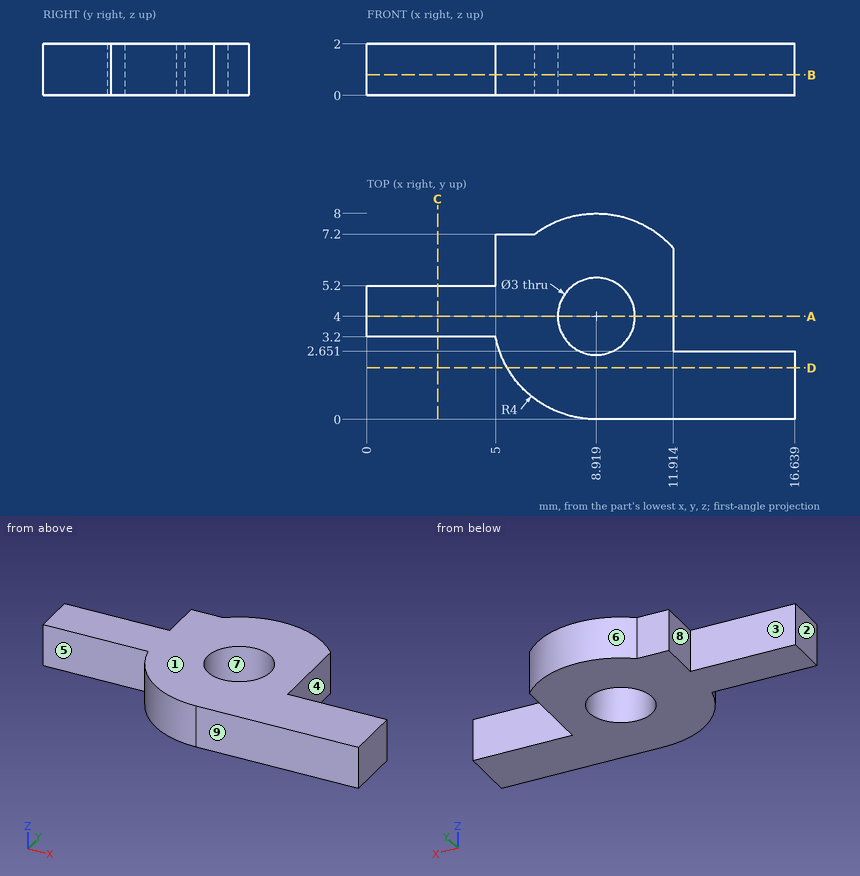
Geometry: see drawing. Coordinates: mm, zero at the bounding-box minimum. A direction names the side the tool comes from. Round coordinates to 2 decimals unless told otherwise and drop trailing zeros. Write each loop counter-clockwise with the first axis right and the second up, starting at its lowest first coordinate (ties: lowest second). Pieces come first, ordered by that corner, then holes.
Item 1: Mould query, pull axis Y, two halves, no side actions, for the marked faces 6, 7, 8 and 9. Classes: +Y half, -Y half, draft (parallel to the pull), parting line (faces both ways), or undercut.
Item 2: Material intervals for L1, parallel to X at y = 6.5, z = 0.75 (1 decimal); L2, parallel to Y at x = 4.75, z = 1.35; L3, parallel to Y at x = 14.25, z = 1.65, sorted ascending.
Item 3: Section query C-C (x = 2.75). Return loops of the section in (y, z).
Item 4: Set-up query: the marked faces 1, 2, 3, 4 and 5. Return all of +Z, -Z, +X, -X, +Y, -Y with unobstructed straight access to the full face (end or side cutting, diameter ignored); none if empty.
Item 5: Section query D-D (y = 2). Return loops of the section in (x, z) (1 decimal).
Item 6: Section query A-A (y = 4). Return loops of the section in (x, z) (1 decimal).
Item 7: Section query B-B (z = 0.8). Return loops of the section in (x, y) (1 decimal).
Item 8: Pin query (flat end, axial travel): P1, Ø0.6, axis at x = 14, z = 1, coming from the +Y side; P2, Ø0.5, axis at x = 5.5, z = 1, coming from the +Y side; P3, Ø1, axis at y = 4.5, z = 1.5, coming from the +X side. Return the tip coordinate at first contact, or that it passes through.
Completed:
1. face 6: +Y half
1. face 7: undercut
1. face 8: draft
1. face 9: -Y half
2. L1: x = 5 to 11.9
2. L2: y = 3.2 to 5.2
2. L3: y = 0 to 2.65
3. outline: (3.2, 0) - (5.2, 0) - (5.2, 2) - (3.2, 2) - close
4. face 1: +Z, +X, -X, +Y, -Y
4. face 2: +Z, -Z, -X, +Y, -Y
4. face 3: +Z, -Z, -X, +Y
4. face 4: +Z, -Z, +X, +Y
4. face 5: +Z, -Z, -X, -Y
5. outline: (5.5, 0) - (16.6, 0) - (16.6, 2) - (5.5, 2) - close
6. outline: (0, 0) - (7.4, 0) - (7.4, 2) - (0, 2) - close; (10.4, 0) - (11.9, 0) - (11.9, 2) - (10.4, 2) - close
7. outline: (0, 3.2) - (5, 3.2) arc R4 ccw to (8.9, 0) - (16.6, 0) - (16.6, 2.7) - (11.9, 2.7) - (11.9, 6.7) arc R4 ccw to (6.5, 7.2) - (5, 7.2) - (5, 5.2) - (0, 5.2) - close; hole circle Ø3 at (8.9, 4)
8. P1: stops at y = 2.65
8. P2: stops at y = 7.2
8. P3: stops at x = 11.91
